Model file for the job. Use its own axes, mm. A direction names the side the tool comes from. Round coordinates to 2 decimals unless told otherwise and drop trailing zeros. Loops run counter-clockwise (first coordinate to the right, second up) from the corner with the lowest first, then second, coordinate; pieces in that order, holes last. Notation, with made-up numbers: M 59.5,-8.5 L 64.5,-8.5 A32 cw 64.5,24.5 Z; hole C -5,42 d10. An arc over 180 degrees is marked long. Answer in a Markdown table with one row per item.
from build123d import *

# Parameters (mm, degrees)
SKETCH1_W           = 35.86
SKETCH1_H           = 17.78
BOSS_EXTRUDE1_DEPTH = 1.6
SKETCH2_W           = 5.5
SKETCH2_H           = 8
BOSS_EXTRUDE2_DEPTH = 2.8
FILLET1_R           = 1


with BuildPart() as part:
    # Sketch1 → Boss-Extrude1 (new body)
    with BuildSketch(Plane(origin=(0, 0, 0), x_dir=(1, 0, 0), z_dir=(0, 1, 0))):
        with Locations((17.93, 8.89)):
            Rectangle(SKETCH1_W, SKETCH1_H)
    extrude(amount=BOSS_EXTRUDE1_DEPTH)

    # Sketch2 → Boss-Extrude2 (add)
    with BuildSketch(Plane(origin=(0, 1.6, 0), x_dir=(1, 0, 0), z_dir=(0, 1, 0))):
        with Locations((2.75, 8.89)):
            Rectangle(SKETCH2_W, SKETCH2_H)
    extrude(amount=BOSS_EXTRUDE2_DEPTH)

    # Fillet1
    fillet1_edges = [part.edges().sort_by_distance(p)[0] for p in [
        (0, 0.8, -17.78),
        (35.86, 0.8, -17.78),
        (35.86, 0.8, 0),
        (0, 0.8, 0),
    ]]
    fillet(fillet1_edges, radius=FILLET1_R)


solid = part.part
1. Saw through at B-B (y = 3.2). Write the cut outline in (x, z).
Verdict:
| item | result |
|---|---|
| outline | M 0,-12.89 L 5.5,-12.89 L 5.5,-4.89 L 0,-4.89 Z |
2. Saw through at A-A (x = 4). Write the cut outline in (y, z), and give its area (3 significant figures).
Verdict:
| item | result |
|---|---|
| outline | M 0,-17.78 L 1.6,-17.78 L 1.6,-12.89 L 4.4,-12.89 L 4.4,-4.89 L 1.6,-4.89 L 1.6,0 L 0,0 Z |
| area | 50.8 mm² |
3. Wall check: probe 1 along Y at (x, z) = (22, -5.25); probe 2 along X at (y, z) = (4, -11.5); probe 3 along Z at (x, y) = (2.5, 3). Give the ranges that are in metal, low to high.
Verdict:
| item | result |
|---|---|
| probe 1 | y = 0 to 1.6 |
| probe 2 | x = 0 to 5.5 |
| probe 3 | z = -12.89 to -4.89 |
4. Pin check, flat tips, straight feed: pin 1 (1.5 mm diameter, centred on x = 30.5, y = 2.5, fed in from +Z); pin 2 (2 mm diameter, centred on x = 1.5, y = 3, fed in from -Z); pin 3 (2 mm diameter, centred on y = 3, z = -10.5, fed in from +X). Stop position of each tip, or through.
Verdict:
| item | result |
|---|---|
| pin 1 | passes through |
| pin 2 | stops at z = -12.89 |
| pin 3 | stops at x = 5.5 |
5. Saw through at C-C (z = -5.75). Write the cut outline in (x, y), and give its area (3 significant figures).
Verdict:
| item | result |
|---|---|
| outline | M 0,0 L 35.86,0 L 35.86,1.6 L 5.5,1.6 L 5.5,4.4 L 0,4.4 Z |
| area | 72.8 mm² |
6. Saw through at D-D (z = -1.75). Write the cut outline in (x, y).
Verdict:
| item | result |
|---|---|
| outline | M 0,0 L 35.86,0 L 35.86,1.6 L 0,1.6 Z |
7. Tool access for faces 1 (the flat face through (5.5, 3, -9)), 2 (the flat face through (3, 3, -12.89)), 3 (the flat face through (3, 3, -4.89)): list every direction of +Z, -Z, +X, -X, +Y, -Y with a clear straight run to the whole face (end or side of a thin tool).
Verdict:
| item | result |
|---|---|
| face 1 | +Z, -Z, +X, +Y |
| face 2 | -Z, +X, -X, +Y |
| face 3 | +Z, +X, -X, +Y |
